Input: part model. Units: mm. Frame: model coordinates. A direction names the side the tool comes from. Give positions to 0.01 mm unless a question says otherwise; leave off trailing zeros. Loops run counter-clockwise (first coordinate to the right, second up) from the corner with the lowest first, then second, coordinate; pieces in that order, holes last. Notation, with made-up numbers: (26, -6) -> (63, -6) arc R20 ccw to (63, 14) -> close; hole circle Ø4 at (82.5, 17.25). An arc over 180 degrees is marked (long way). Answer as a JSON object with one key per item and string values.
```python
from build123d import *

# Parameters (mm, degrees)
F0_R     = 66
F0_R_2   = 17.5
F0_R_3   = 7.5
F1_DEPTH = 10
F2_DEPTH = 18
F3_R     = 5
F3_R_2   = 4.25
F3_R_3   = 4
F4_DEPTH = 10


with BuildPart() as f1:
    # F0 (on Top) → F1 (new body)
    with BuildSketch(Plane.XY):
        Circle(F0_R)
        Circle(F0_R_2, mode=Mode.SUBTRACT)
        Circle(F0_R_2)
        Circle(F0_R_3, mode=Mode.SUBTRACT)
    extrude(amount=F1_DEPTH)

    # F0 (on Top) → F2 (join)
    with BuildSketch(Plane.XY):
        Circle(F0_R_2)
        Circle(F0_R_3, mode=Mode.SUBTRACT)
    extrude(amount=F2_DEPTH)

    # F3 (on face) → F4 (cut, through all)
    with BuildSketch(Plane.XY.offset(10)):
        with Locations((0, -25)):
            Circle(F3_R)
        with Locations((21.650635, 12.5)):
            Circle(F3_R)
        with Locations((0, 25)):
            Circle(F3_R)
        with Locations((-21.650635, 12.5)):
            Circle(F3_R)
        with Locations((-33, 0)):
            Circle(F3_R)
        with Locations((33, 0)):
            Circle(F3_R)
        with Locations((-34.641016, -20)):
            Circle(F3_R_2)
        with Locations((0, 40)):
            Circle(F3_R_2)
        with Locations((34.641016, -20)):
            Circle(F3_R_2)
        with Locations((0, -55)):
            Circle(F3_R_3)
        with Locations((-47.631397, 27.5)):
            Circle(F3_R_3)
        with Locations((47.631397, 27.5)):
            Circle(F3_R_3)
    extrude(amount=-F4_DEPTH, mode=Mode.SUBTRACT)


solid = f1.part
```
Q1. Section A-A, the plane x = 0. Return the cut outline in (y, z), then the cut area to 3 significant figures.
Evaluation:
{"outline": "(-66, 0) -> (-59, 0) -> (-59, 10) -> (-66, 10) -> close; (-51, 0) -> (-30, 0) -> (-30, 10) -> (-51, 10) -> close; (-20, 0) -> (-7.5, 0) -> (-7.5, 18) -> (-17.5, 18) -> (-17.5, 10) -> (-20, 10) -> close; (7.5, 0) -> (20, 0) -> (20, 10) -> (17.5, 10) -> (17.5, 18) -> (7.5, 18) -> close; (30, 0) -> (35.75, 0) -> (35.75, 10) -> (30, 10) -> close; (44.25, 0) -> (66, 0) -> (66, 10) -> (44.25, 10) -> close", "area": "965 mm2"}
Q2. Draft query along Y for faces 3 (the flat face through (14, 1, 0)), 4 (the cylindrical face through (-1.08, 20.12, 5.07)), 5 (the cylindrical face through (-13.887, -10.648, 13.944)), 6 (the cylindrical face through (28, 0, 5)). Return one class per face: +Y half, -Y half, draft (parallel to the pull), parting line (faces both ways), or undercut.
Evaluation:
{"face 3": "draft", "face 4": "undercut", "face 5": "parting line", "face 6": "undercut"}
Q3. Section B-B, the plane z = 3. Give the number of separate pieces and of enclosed holes in the cut face, then the cut area to 3 significant figures.
Evaluation:
{"separate pieces": "1", "enclosed holes": "13", "area": "12,700 mm2"}
Q4. Section C-C, the plane y = 40. Return the cut outline in (x, z), then the cut area to 3 significant figures.
Evaluation:
{"outline": "(-52.5, 0) -> (-4.25, 0) -> (-4.25, 10) -> (-52.5, 10) -> close; (4.25, 0) -> (52.5, 0) -> (52.5, 10) -> (4.25, 10) -> close", "area": "965 mm2"}
Q5. Section D-D, the plane x = -49. Return the cut outline in (y, z), then the cut area to 3 significant figures.
Evaluation:
{"outline": "(-44.22, 0) -> (23.74, 0) -> (23.74, 10) -> (-44.22, 10) -> close; (31.26, 0) -> (44.22, 0) -> (44.22, 10) -> (31.26, 10) -> close", "area": "809 mm2"}
Q6. Pin query (flat end, axial travel): pin 1 (5 mm diameter, centred on x = -47.63, y = 27.5, fed in from -Z); pin 2 (10 mm diameter, centred on x = -31, y = -41.5, fed in from +Z); pin 3 (13 mm diameter, centred on x = 0, y = -55, fed in from -Z); pin 4 (10 mm diameter, centred on y = -25, z = 9, fed in from -X). Return the tip coordinate at first contact, or that it passes through.
Evaluation:
{"pin 1": "passes through", "pin 2": "stops at z = 10", "pin 3": "stops at z = 0", "pin 4": "stops at x = -62.9"}
Q7. Access query for faces 1 (the flat face through (14, -14, 10)), 2 (the cylindrical face through (-16.88, 14, 5.07)). Directions: +Z, -Z, +X, -X, +Y, -Y. A direction counts if a zero-diameter tool reaches every point of the face in a straight line with its end or side. Return the directions, or none.
Evaluation:
{"face 1": "+Z", "face 2": "+Z, -Z"}
Q8. Ray query, line 1 along Y through (x, z) = (0, 6.5); line 2 along Y through (x, z) = (-31.5, 1.75); line 3 along Z through (x, y) = (4, 56). Return the intervals inside material, ascending.
Evaluation:
{"line 1": "y = -66 to -59, -51 to -30, -20 to -7.5, 7.5 to 20, 30 to 35.75, 44.25 to 66", "line 2": "y = -58 to -22.86, -17.14 to -4.77, 4.77 to 58", "line 3": "z = 0 to 10"}
